Geometry: final body of the model. Coordinates: model frame, mm. A direction names the side the tool comes from. Coordinates: 2 decimals unless noted, no trailing zeros. Order: outer loops, then holes, each group sorted by start corner. A loop starts at its lowest first (then second) coordinate and runs counter-clockwise, first axis right, second up. Notation, with made-up numbers: (-24.75, -18) -> (2.25, -18) arc R26 cw to (2.25, 3) -> close; hole circle Ø10 at (20, 54). An arc over 180 degrees is marked (long way). Answer in a Markdown table with one row per item. Add a question column.
1) Section query C-C on y = 1.85. Return the cut outline in (x, z) (1 decimal), then the cut area to 3 significant figures.
2) Pull-direction query (Z, two-part tool) for faces 1 (the face through (-1.588, 2, 0)), 2 (the face through (3.175, 2, -9)), 3 (the face through (0, 2, -7.938)), 4 (the face through (1.588, 2, 0)); classes: +Z half, -Z half, draft (parallel to the pull), parting line (faces both ways), or undercut.
3) Contact query for flat-ended pins moving along their axis: P1, Ø0.9, axis at y = 2, z = 9.5, coming from the -X side; P2, Ø1, axis at x = -1, y = 2, coming from the -Z side; P3, Ø1.6, axis at y = 1.5, z = -1, coming from the -X side. Output: stop coordinate, or through.
4) Section query A-A on x = 0. Return the cut outline in (y, z) (1 decimal).
5) Set-up query: faces 5 (the face through (-4.762, 2, -7)), 6 (the face through (-4, 2, 10.897)), 7 (the face through (-0.035, 1.61, -4.762)), 8 (the face through (-3.175, 2, -9)), 9 (the face through (0, 2, 7.938)). Return all of +Z, -Z, +X, -X, +Y, -Y with unobstructed straight access to the full face (end or side cutting, diameter ignored); none if empty.
6) Ray query, line 1 (X direction, y = 1.7, z = 8) (1 decimal); line 2 (X direction, y = 0.2, z = -7.75); line 3 (Z direction, x = -2.25, y = 1.95). Return the intervals inside material, ascending. Write a range as from..to.
7) Section query B-B on z = 8.75. Return the cut outline in (x, y) (1 decimal).
8) Section query D-D on x = -6. Return the cut outline in (y, z) (3 decimals), then the cut area to 3 significant figures.
```python
from build123d import *

# Parameters (mm, degrees)
BOSS_EXTRUDE1_DEPTH = 3.175
CUT_EXTRUDE1_REACH  = 5.175


with BuildPart() as part:
    # Sketch2 → Boss-Extrude1 (new body)
    with BuildSketch(Plane(origin=(0, 0, 0), x_dir=(1, 0, 0), z_dir=(0, 1, 0))):
        with BuildLine():
            Line((-3.175, 10.8966), (-3.175, 7.9375))
            Line((-3.175, 7.9375), (3.175, 7.9375))
            Line((3.175, 7.9375), (3.175, 10.8966))
            Line((3.175, 10.8966), (4.7625, 10.8966))
            Line((4.7625, 10.8966), (4.7625, -10.8966))
            Line((4.7625, -10.8966), (3.175, -10.8966))
            Line((3.175, -10.8966), (3.175, -7.9375))
            Line((3.175, -7.9375), (-3.175, -7.9375))
            Line((-3.175, -7.9375), (-3.175, -10.8966))
            Line((-3.175, -10.8966), (-4.7625, -10.8966))
            Line((-4.7625, -10.8966), (-4.7625, -2.33313898))
            ThreePointArc((-4.7625, -2.33313898), (-6.6675, 0), (-4.7625, 2.33313898))
            Line((-4.7625, 2.33313898), (-4.7625, 10.8966))
            Line((-4.7625, 10.8966), (-3.175, 10.8966))
        make_face()
    extrude(amount=BOSS_EXTRUDE1_DEPTH)

    # Sketch3 → Cut-Extrude1 (cut, up to next)
    with BuildSketch(Plane(origin=(0, 3.175, 0), x_dir=(1, 0, 0), z_dir=(0, 1, 0)), mode=Mode.PRIVATE) as cut_extrude1_sk1:
        with BuildLine():
            Line((1.5875, 3.175), (1.5875, -3.175))
            ThreePointArc((1.5875, -3.175), (0, -4.7625), (-1.5875, -3.175))
            Line((-1.5875, -3.175), (-1.5875, 3.175))
            ThreePointArc((-1.5875, 3.175), (0, 4.7625), (1.5875, 3.175))
        make_face()
    cut_extrude1_tool1 = extrude(cut_extrude1_sk1.sketch, amount=-CUT_EXTRUDE1_REACH, mode=Mode.PRIVATE) & part.part
    add(cut_extrude1_tool1.solids().sort_by_distance((0, 3.175, 0))[0], mode=Mode.SUBTRACT)


solid = part.part
```
Result:
| question | item | result |
|---|---|---|
| 1 | outline | (-4.8, -10.9) -> (-3.2, -10.9) -> (-3.2, -7.9) -> (3.2, -7.9) -> (3.2, -10.9) -> (4.8, -10.9) -> (4.8, 10.9) -> (3.2, 10.9) -> (3.2, 7.9) -> (-3.2, 7.9) -> (-3.2, 10.9) -> (-4.8, 10.9) -> (-4.8, 2.3) arc R2.4 ccw to (-4.8, -2.3) -> close; hole (-1.6, -3.2) arc R1.6 ccw to (1.6, -3.2) -> (1.6, 3.2) arc R1.6 ccw to (-1.6, 3.2) -> close |
| 1 | area | 149 mm2 |
| 2 | face 1 | undercut |
| 2 | face 2 | draft |
| 2 | face 3 | -Z half |
| 2 | face 4 | undercut |
| 3 | P1 | x = -4.76 |
| 3 | P2 | z = -7.94 |
| 3 | P3 | x = -6.66 |
| 4 | outline | (0, -7.9) -> (3.2, -7.9) -> (3.2, -4.8) -> (0, -4.8) -> close; (0, 4.8) -> (3.2, 4.8) -> (3.2, 7.9) -> (0, 7.9) -> close |
| 5 | face 5 | -Z, -X, +Y, -Y |
| 5 | face 6 | +Z, +X, -X, +Y, -Y |
| 5 | face 7 | +Y, -Y |
| 5 | face 8 | -Z, +Y, -Y |
| 5 | face 9 | +Z, +Y, -Y |
| 6 | line 1 | -4.8..-3.2, 3.2..4.8 |
| 6 | line 2 | -4.76..4.76 |
| 6 | line 3 | -7.94..7.94 |
| 7 | outline | (-4.8, 0) -> (-3.2, 0) -> (-3.2, 3.2) -> (-4.8, 3.2) -> close; (3.2, 0) -> (4.8, 0) -> (4.8, 3.2) -> (3.2, 3.2) -> close |
| 8 | outline | (0, -1.653) -> (3.175, -1.653) -> (3.175, 1.653) -> (0, 1.653) -> close |
| 8 | area | 10.5 mm2 |
